```python
from build123d import *

# Parameters (mm, degrees)
SKETCH1_R           = 1.610492359
SKETCH1_R_2         = 1.59089725
SKETCH1_R_3         = 1.6
SKETCH1_W           = 222.015696088
SKETCH1_H           = 125.972340976
BOSS_EXTRUDE1_DEPTH = 3


with BuildPart() as part:
    # Sketch1 → Boss-Extrude1 (new body)
    with BuildSketch(Plane.XY):
        with BuildLine():
            Line((-105.5, -74.342560363), (-8.826077226, -74.342560363))
            ThreePointArc((-8.826077226, -74.342560363), (-8.626849156, -74.301174008), (-8.460609358, -74.183832695))
            ThreePointArc((-8.460609358, -74.183832695), (-7.882511931, -73.28221691), (-7.661371157, -72.234264423))
            Line((-7.661371157, -72.234264423), (-7.660812811, -71.693665015))
            ThreePointArc((-7.660812811, -71.693665015), (-7.514183841, -71.340445506), (-7.160813078, -71.194181429))
            Line((-7.160813078, -71.194181429), (7.839186922, -71.194181429))
            ThreePointArc((7.839186922, -71.194181429), (8.192557686, -71.340445506), (8.339186655, -71.693665015))
            Line((8.339186655, -71.693665015), (8.338670775, -72.154345161))
            ThreePointArc((8.338670775, -72.154345161), (8.546458509, -73.246362553), (9.140780516, -74.185755485))
            ThreePointArc((9.140780516, -74.185755485), (9.288714604, -74.294526792), (9.465938947, -74.342560363))
            Line((9.465938947, -74.342560363), (105.5, -74.342560363))
            ThreePointArc((105.5, -74.342560363), (106.914213562, -74.928346801), (107.5, -76.342560363))
            Line((107.5, -76.342560363), (107.5, -77.588833763))
            ThreePointArc((107.5, -77.588833763), (108.085786438, -79.003047325), (109.5, -79.588833763))
            Line((109.5, -79.588833763), (119.500003053, -79.588833763))
            Line((119.500003053, -79.588833763), (119.500003053, -78.888833763))
            Line((119.500003053, -78.888833763), (119.500003053, 79.91034623))
            ThreePointArc((119.500003053, 79.91034623), (118.912699712, 81.328214854), (117.494826949, 81.9155082))
            Line((117.494826949, 81.9155082), (-117.5, 81.913851764))
            ThreePointArc((-117.5, 81.913851764), (-118.914213562, 81.328065327), (-119.5, 79.913851764))
            Line((-119.5, 79.913851764), (-119.5, 0))
            Line((-119.5, 0), (-119.5, -78.888833763))
            Line((-119.5, -78.888833763), (-119.5, -79.588833763))
            Line((-119.5, -79.588833763), (-109.5, -79.588833763))
            ThreePointArc((-109.5, -79.588833763), (-108.085786438, -79.003047325), (-107.5, -77.588833763))
            Line((-107.5, -77.588833763), (-107.5, -76.342560363))
            ThreePointArc((-107.5, -76.342560363), (-106.914213562, -74.928346801), (-105.5, -74.342560363))
        make_face()
        with Locations((-113.5, -73.988833763)):
            Circle(SKETCH1_R, mode=Mode.SUBTRACT)
        with Locations((113.5, -73.988833763)):
            Circle(SKETCH1_R_2, mode=Mode.SUBTRACT)
        with Locations((-113.5, 77.014278693)):
            Circle(SKETCH1_R_3, mode=Mode.SUBTRACT)
        with Locations((0.009179053, 1.722083042)):
            Rectangle(SKETCH1_W, SKETCH1_H, mode=Mode.SUBTRACT)
        with Locations((113.5, 77.011166237)):
            Circle(SKETCH1_R_3, mode=Mode.SUBTRACT)
    extrude(amount=BOSS_EXTRUDE1_DEPTH)


solid = part.part
```
CAD build for the part. Positions are in the model's coordinates, mm. Give positions to 0.01 mm unless a question says otherwise; leave off trailing zeros. Write each loop counter-clockwise with the first axis right and the second up, starting at its lowest first coordinate (ties: lowest second). Pieces come first, ordered by that corner, then holes. Notation, with made-up numbers: M 36,56.5 L 58,56.5 A25 cw 58,88.5 Z; hole C 49,6 d10. An arc over 180 degrees is marked long. Return JSON: item names as keys, results as strings. Group by question number.
(1) Band-saw the part on A-A (y = 16). Give the cut face in (x, z).
(2) Band-saw the part on C-C (z = 1.8). State how many separate pieces and enclosed holes the cut face has, and give its area (3 significant figures).
(3) Band-saw the part on B-B (x = -97). Give the cut face in (y, z), and give its area (3 significant figures).
(4) Drill centre lines: L1, parallel to Y at x = 113.5, z = 1.3; L2, parallel to Y at x = 56, z = 1.6; L3, parallel to X at y = 52, z = 2.95. Where is each one in solid material? Low to high. Write a range as [from, to].
(5) Flat gauge pins, fed straight in: pin 1 Ø0.9 at (x, z) = (52.5, 1) entering from -Y; pin 2 Ø2.5 at (x, y) = (113.5, -73.99) entering from -Z; pin 3 Ø4 at (x, y) = (-113.5, -73.99) entering from +Z. Where does each tip first touch, or does it go through?
Entries:
{
 "1": {"outline": "M -119.5,0 L -111,0 L -111,3 L -119.5,3 Z; M 111.02,0 L 119.5,0 L 119.5,3 L 111.02,3 Z"},
 "2": {"separate pieces": "1", "enclosed holes": "5", "area": "9,420 mm^2"},
 "3": {"outline": "M -74.34,0 L -61.26,0 L -61.26,3 L -74.34,3 Z; M 64.71,0 L 81.91,0 L 81.91,3 L 64.71,3 Z", "area": "90.9 mm^2"},
 "4": {"L1": "y = [-79.59, -75.58], [-72.4, 75.41], [78.61, 81.92]", "L2": "y = [-74.34, -61.26], [64.71, 81.92]", "L3": "x = [-119.5, -111], [111.02, 119.5]"},
 "5": {"pin 1": "stops at y = -74.34", "pin 2": "passes through", "pin 3": "stops at z = 3"}
}
